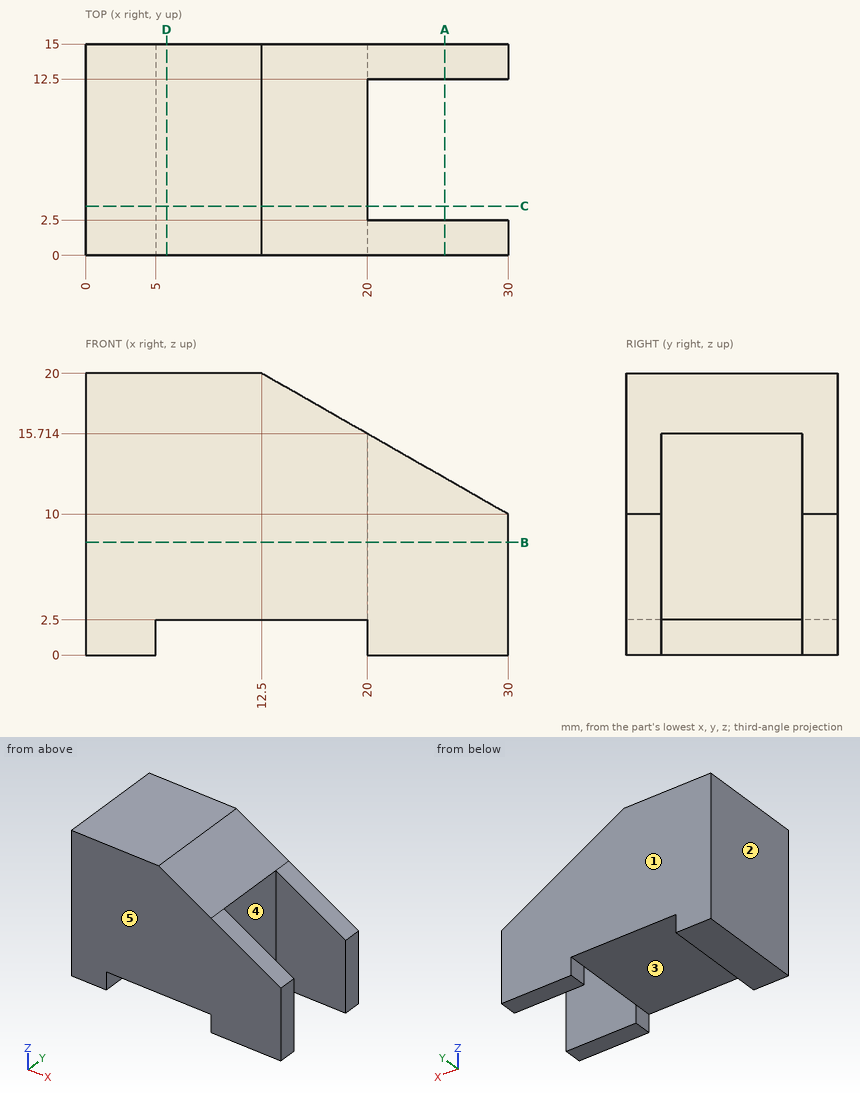
Geometry check sheet. Reference: drawing and pictorial views, mm from the part's lowest x, y, z. A direction names the side the tool comes from. Give positions to 0.01 mm unless a question says otherwise; leave off trailing zeros. Loops run counter-clockwise (first coordinate to the right, second up) from the corner with the lowest first, then second, coordinate; pieces in that order, holes last.
1. Thickness scan on line 1 (X direction, y = 2.75, z = 5.25); line 2 (Z direction, x = 9.5, y = 11.5); line 3 (Y direction, x = 26.75, z = 9.25). Record the ranges inside material, lowest first.
2. Set-up check for the marked faces 4 and 5: record each of +Z, -Z, +X, -X, +Y, -Y from which the full face is reachable in a straight line by a thin tool's end or side.
3. Section check B-B, the plane z = 8. Enter the section's corners in (x, y), then the cut area to 3 significant figures.
4. Go/stop test with flat-tipped pins: pin 1 Ø1 at (y, z) = (8.5, 14.5) entering from +X; pin 2 Ø2 at (x, y) = (25, 1.5) entering from +Z; pin 3 Ø4 at (x, z) = (21, 17.5) entering from +Y. Record where each tip stops, or that it passes through.
5. Section check D-D, the plane x = 5.75. Enter the section's corners in (y, z), then the cut area to 4 significant figures.
6. Section check C-C, the plane y = 3.5. Enter the section's corners in (x, z).
7. Mould release check, pull along X, two halves, no side actions. Record for the marked faces 1, 2 and 3: released by +X, released by -X, zero draft, split by the parting line, or undercut.
8. Section check A-A, the plane x = 25.5. Enter the section's corners in (y, z).
Geometry says:
1. line 1: x = 0 to 20
1. line 2: z = 2.5 to 20
1. line 3: y = 0 to 2.5, 12.5 to 15
2. face 4: +Z, -Z, +X
2. face 5: +Z, -Z, +X, -X, -Y
3. outline: (0, 0) - (30, 0) - (30, 2.5) - (20, 2.5) - (20, 12.5) - (30, 12.5) - (30, 15) - (0, 15) - close
3. area: 350 mm2
4. pin 1: stops at x = 20
4. pin 2: stops at z = 13.43
4. pin 3: passes through
5. outline: (0, 2.5) - (15, 2.5) - (15, 20) - (0, 20) - close
5. area: 262.5 mm2
6. outline: (0, 0) - (5, 0) - (5, 2.5) - (20, 2.5) - (20, 15.71) - (12.5, 20) - (0, 20) - close
7. face 1: zero draft
7. face 2: released by -X
7. face 3: undercut
8. outline: (0, 0) - (2.5, 0) - (2.5, 12.57) - (0, 12.57) - close; (12.5, 0) - (15, 0) - (15, 12.57) - (12.5, 12.57) - close
